Autodesk Inventor part; units mm, degrees
ref_plane "Start Plane" through (0, 0, 0) normal (0, 0, 1) x (1, 0, 0)
ref_plane "End Plane" through (0, 0, 1306.5) normal (0, 0, 1) x (1, 0, 0)
ref_plane "Work Plane5" through (-200, 9, 1306.5) normal (0, 0, 1) x (1, 0, 0)
ref_plane "Start Plane" through (0, 0, 0) normal (0, 0, 1) x (1, 0, 0)
ref_plane "End Plane" through (0, 0, 1306.5) normal (0, 0, 1) x (1, 0, 0)
sketch "Sketch" plane through (0, 0, 0) normal (0, 0, 1) x (1, 0, 0)
  line L0 (-15, -9) -> (-15, 9)
  line L1 (-9, 15) -> (9, 15)
  line L2 (15, 9) -> (15, -9)
  line L3 (9, -15) -> (-9, -15)
  arc A0 (-15, -9) -> (-9, -15) centre (-9, -9) ccw
  arc A1 (-9, 15) -> (-15, 9) centre (-9, 9) ccw
  arc A2 (15, 9) -> (9, 15) centre (9, 9) ccw
  arc A3 (9, -15) -> (15, -9) centre (9, -9) ccw
  arc A4 (-9, 12) -> (-12, 9) centre (-9, 9) ccw
  line L4 (-9, 12) -> (9, 12)
  arc A5 (12, 9) -> (9, 12) centre (9, 9) ccw
  line L5 (12, 9) -> (12, -9)
  arc A6 (9, -12) -> (12, -9) centre (9, -9) ccw
  line L6 (9, -12) -> (-9, -12)
  arc A7 (-12, -9) -> (-9, -12) centre (-9, -9) ccw
  line L7 (-12, -9) -> (-12, 9)
  line L8 (0, 22.7397) -> (0, -22.7397) construction
  line L9 (-22.7397, 0) -> (22.7397, 0) construction
  dimension "d7" = 6
  dimension "d10" = 30
  dimension "d11" = 30
  dimension "d12" = 3
  dimension "d15" = 15
  dimension "d16" = 15
extrude "Body" add sketch "Sketch" along normal up to surface (1306.5 mm away) from surface at 0
sketch "Sketch3" plane through (0, 0, 0) normal (0, 0, 1) x (1, 0, 0)
  line L0 (0, 0) -> (10, 0)
ref_plane "Work Plane3" through (0, 0, 0) normal (0, -1, 0) x (1, 0, 0)
ref_plane "Work Plane5" through (-200, 9, 1306.5) normal (0, 0, 1) x (1, 0, 0)
split "Split2" plane through (-200, 9, 1306.5) removes the side toward (0, 0, 1)
sketch "Sketch4" plane through (0, 0, 0) normal (0, -1, 0) x (1, 0, 0)
  line L0 (-2, 0) -> (12, 0)
  line L1 (-2, 1306.5) -> (12, 1306.5)
  dimension "d18" = 1306.5
equation "\"d7\" = G_IR"
equation "\"d10\" = G_H"
equation "\"d11\" = G_W"
equation "\"d12\" = G_T"
equation "\"d15\" = 0.5 * d10"
equation "\"d16\" = 0.5 * d11"
equation "\"d3\" = G_L"
equation "\"G_W\" = 30"
equation "\"G_H\" = 30"
equation "\"G_T\" = 3"
equation "\"G_IR\" = 6"
equation "\"G_L\" = d18"
equation "\"G_OFFSET_START\" = 0"
equation "\"G_OFFSET_END\" = -15"
equation "\"d14\" = G_OFFSET_END + B_L"
equation "\"B_L\" = 1321.5"
properties part number "DIN EN 10219-2 - 30 x 30 x 3  - 1306.5" material "Steel, Mild"
The model under review builds one solid part; all positions refer to its coordinate system, in mm. Give positions to 0.01 mm unless a question says otherwise; leave off trailing zeros. Write each loop counter-clockwise with the first axis right and the second up, starting at its lowest first coordinate (ties: lowest second). Pieces come first, ordered by that corner, then holes.
(1) To check wall thickness, follow L1, parallel to Y at x = 8.5, z = 1002; L2, parallel to X at y = -11.75, z = 1051.5. State the ranges of each line that lie inside material, in increasing order.
(2) For P1, Ø1, axis at y = -11.5, z = 421.5, coming from the +X side, flat-tipped, find the tip position at first contact; note if it passes through.
(3) Consider section A-A, the plane x = 0. Give the boundary of the cut face in (y, z).
(4) Consider section B-B, the plane z = 121. Give the boundary of the cut face in (x, y).
Returned:
1. L1: y = -15 to -12, 12 to 15
1. L2: x = -14.33 to -10.2, 10.2 to 14.33
2. P1: stops at x = 14.66
3. outline: (-15, 0) - (-12, 0) - (-12, 1306.5) - (-15, 1306.5) - close; (12, 0) - (15, 0) - (15, 1306.5) - (12, 1306.5) - close
4. outline: (-15, -9) arc R6 ccw to (-9, -15) - (9, -15) arc R6 ccw to (15, -9) - (15, 9) arc R6 ccw to (9, 15) - (-9, 15) arc R6 ccw to (-15, 9) - close; hole (-12, -9) arc R3 ccw to (-9, -12) - (9, -12) arc R3 ccw to (12, -9) - (12, 9) arc R3 ccw to (9, 12) - (-9, 12) arc R3 ccw to (-12, 9) - close
